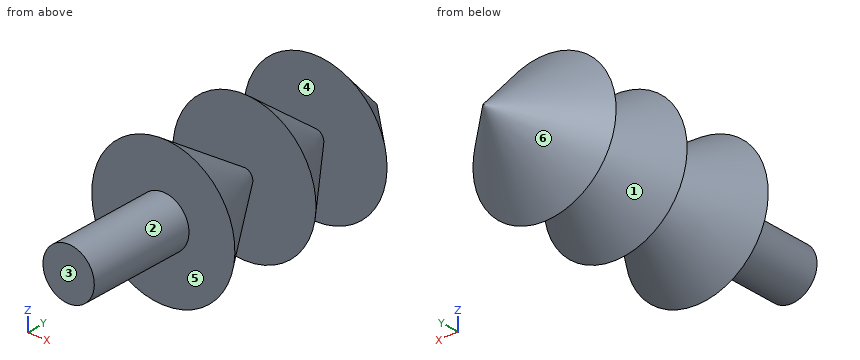
```python
from build123d import *

# Parameters (mm, degrees)
SKETCH_1_R      = 8
EXTRUDE_1_DEPTH = 40


with BuildPart() as part:
    # 草图1 → 凸台-拉伸1 (new body)
    with BuildSketch(Plane(origin=(0, 0, 0), x_dir=(1, 0, 0), z_dir=(0, 1, 0))):
        with Locations(Location((0, 0, 0), (0, 0, 270))):
            Circle(SKETCH_1_R)
    extrude(amount=EXTRUDE_1_DEPTH)

    # 草图2 → 切除-旋转1 (revolve, cut)
    with BuildSketch(Plane(origin=(0, 0, 0), x_dir=(0, 0, -1), z_dir=(1, 0, 0)), mode=Mode.PRIVATE) as cut_revolve_1_sk:
        Polygon((-0.055370982, 40), (-8, 32.055370982), (-0.935929442, 32.055370982), (-8, 22.83286128), (-0.935929442, 22.83286128), (-8, 12.295716869), (-2.86773925, 12.295716869), (-2.86773925, -1.226951792), (-16.741646059, 0.704858016), (-12.965835978, 40), (-8.83878775, 42.326578441), align=None)
    revolve(cut_revolve_1_sk.sketch.rotate(Axis((0, 40, 0), (0, -1, 0)), 180), axis=Axis((0, 40, 0), (0, -1, 0)), mode=Mode.SUBTRACT)


solid = part.part
```
Design review of the part built by this model. Coordinates are the model's own, in mm. Face numbers are marked on the shaded views. A direction names the side the tool comes from. Give positions to 0.01 mm unless a question says otherwise; leave off trailing zeros. Order: outer loops, then holes, each group sorted by start corner. A loop starts at its lowest first (then second) coordinate and runs counter-clockwise, first axis right, second up. Notation, with made-up numbers: M 68.5,49.25 L 78.5,49.25 A16 ccw 78.5,70.25 Z; hole C -1,42 d2. An arc over 180 degrees is marked long. One line per question, with ' | ' between items. Start each with the question number.
Q1. For pin 1 Ø3 at (x, z) = (-5, 1) entering from +Y; pin 2 Ø1.5 at (y, z) = (12, -1) entering from -X; pin 3 Ø1 at (y, z) = (17.5, -1.5) entering from +X, all flat-tipped, find the tip position at first contact; note any pin that passes through.
Q2. We need section D-D (y = 35.5). Write out the cut boundary in (x, z), plus the area to 3 significant figures.
Q3. For L1, parallel to Y at x = 3.75, z = -1.25; L2, parallel to Y at x = 1.5, z = 1.25; L3, parallel to Z at x = 5.25, y = 12.5, list the stretches that pass through material, from the lowest coordinate up. Write a range as [from, to].
Q4. We need section A-A (z = -2.25). State how many separate pieces and enclosed holes the cut face has, plus the area to 3 significant figures.
Q5. We need section C-C (y = 21). Write out the cut boundary in (x, z), plus the area to 3 significant figures.
Q6. The part is to be moulded in two halves that separate along Y. For the marked faces 4, 5 and 6, say which applies: +Y half, -Y half, draft (parallel to the pull), parting line (faces both ways), or undercut.
Q7. Machinability: for the marked faces 1, 2 and 3, which of the approach directions +Z, -Z, +X, -X, +Y, -Y give a long, thin tool a straight path to every point of the face, cutting with its end or side? Answer none if there is none.
Returned:
1) pin 1: y = 36.46 | pin 2: x = -7.99 | pin 3: x = 4.64
2) outline: C 0,0 d9.11 | area: 65.2 mm2
3) L1: [12.3, 18.33], [22.83, 28.12], [32.06, 36.1] | L2: [0, 21.32], [22.83, 30.73], [32.06, 38.1] | L3: [-5.85, 5.85]
4) separate pieces: 3 | enclosed holes: 0 | area: 240 mm2
5) outline: C 0,0 d4.33 | area: 14.7 mm2
6) face 4: undercut | face 5: -Y half | face 6: +Y half
7) face 1: none | face 2: -Y | face 3: +Z, -Z, +X, -X, -Y
